Input: part model. Units: mm. Frame: model coordinates. A direction names the side the tool comes from. Give positions to 0.01 mm unless a question says otherwise; leave off trailing zeros. Order: outer loops, then holes, each group sorted by start corner. A loop starts at its lowest first (then second) coordinate and runs counter-clockwise, first axis right, second up. Notation, with made-up numbers: (-10.75, 43.25) - (8.25, 43.25) arc R19 ccw to (8.25, 60.25) - close; hole circle Ø6 at (-22.5, 83.25). An arc over 180 degrees is marked (long way). Answer in a Markdown table with one row per item. Add a question column.
1. Contact query for flat-ended pins moving along their axis: pin 1 (5.5 mm diameter, centred on x = -14.8, y = -14.8, fed in from -Z); pin 2 (10 mm diameter, centred on x = -7.5, z = -14.5, fed in from -Y); pin 3 (2 mm diameter, centred on x = 1.5, y = -8.5, fed in from +Z); pin 4 (0.5 mm diameter, centred on y = 5.5, z = 41, fed in from -X). Output: stop coordinate, or through.
2. Mould query, pull axis Y, two halves, no side actions, for faces 4 (the face through (0, 4.561, 36)), 5 (the face through (18.1, -18.14, 6.12)), 6 (the face through (16.9, 14.89, -29.26)). Classes: released by +Y, released by -Y, zero draft, split by the parting line, or undercut.
3. Access query for faces 1 (the face through (10.55, -15, 14)), 2 (the face through (-12, 14, 12.065)), 3 (the face through (1.588, 5, 37)). Directions: +Z, -Z, +X, -X, +Y, -Y. A direction counts if a zero-diameter tool reaches every point of the face in a straight line with its end or side. Return the directions, or none.
4. Section query D-D on y = 8. Return loops of the section in (x, z), and give its area (3 significant figures).
5. Section query A-A on x = 14.8. Count the separate pieces of the cut face and the enclosed holes in it, and give its area (3 significant figures).
6. Section query C-C on z = 47. Return loops of the section in (x, y), and give its area (3 significant figures).
7. Ray query, line 1 (X direction, y = -14.8, z = 5.25); line 2 (Y direction, x = 14.8, z = -27.75). Return the intervals inside material, ascending. Write a range as [from, to].
```python
from build123d import *

# Parameters (mm, degrees)
SKETCH1_W                      = 38.1
SKETCH1_H                      = 38.1
EXTRUDE1_DEPTH                 = 15.24
FILLET1_R                      = 3.175
SKETCH2_R                      = 6.35
EXTRUDE2_DEPTH                 = 38.1
CHAMFER1_SIZE                  = 1
SKETCH3_W                      = 3.175
SKETCH3_H                      = 3.175
EXTRUDE3_DEPTH                 = 35
FILLET2_R                      = 1.5875
M5X0_8_TAPPED_HOLE1_D          = 4.2
M5X0_8_TAPPED_HOLE1_DEPTH      = 14
M5X0_8_TAPPED_HOLE1_TIP        = 1.2618073
SKETCH7_R                      = 18.5
EXTRUDE4_DEPTH                 = 25.4
EXTRUDE5_DEPTH                 = 7.62
SKETCH9_W                      = 8.5
SKETCH9_H                      = 8.5
EXTRUDE7_DEPTH                 = 3.175
FILLET3_R                      = 1.5
SKETCH10_R                     = 2.5
EXTRUDE8_DEPTH                 = 12.065
M5X0_8_TAPPED_HOLE2_D          = 4.2
M5X0_8_TAPPED_HOLE3_AT_2_COUNT = 2
M5X0_8_TAPPED_HOLE3_AT_2_PITCH = 19.05
M5X0_8_TAPPED_HOLE3_AT_3_COUNT = 2
M5X0_8_TAPPED_HOLE3_AT_3_PITCH = 36.83
M5X0_8_TAPPED_HOLE3_AT_4_COUNT = 2
M5X0_8_TAPPED_HOLE3_AT_4_PITCH = 41.465062402


with BuildPart() as part:
    # Sketch1 → Extrude1 (new body)
    with BuildSketch(Plane.XY):
        Rectangle(SKETCH1_W, SKETCH1_H)
    extrude(amount=EXTRUDE1_DEPTH)

    # Fillet1
    fillet1_edges = [part.edges().sort_by_distance(p)[0] for p in [
        (19.05, -19.05, 7.62),
        (-19.05, -19.05, 7.62),
        (-19.05, 19.05, 7.62),
        (19.05, 19.05, 7.62),
    ]]
    fillet(fillet1_edges, radius=FILLET1_R)

    # Sketch2 → Extrude2 (add)
    with BuildSketch(Plane.XY.offset(15.24)):
        with Locations(Location((0, 0, 0), (0, 0, 180))):
            Circle(SKETCH2_R)
    extrude(amount=EXTRUDE2_DEPTH)

    # Chamfer1
    chamfer1_edges = [part.edges().sort_by_distance(p)[0] for p in [
        (6.35, 0, 53.34),
    ]]
    chamfer(chamfer1_edges, length=CHAMFER1_SIZE)

    # Sketch3 → Extrude3 (cut)
    with BuildSketch(Plane.XY.offset(53.34)):
        with Locations((0, 6.148361062)):
            Rectangle(SKETCH3_W, SKETCH3_H)
    extrude(amount=-EXTRUDE3_DEPTH, mode=Mode.SUBTRACT)

    # Fillet2
    fillet2_edges = [part.edges().sort_by_distance(p)[0] for p in [
        (1.5875, 5.354611062, 18.34),
        (-1.5875, 5.354611062, 18.34),
    ]]
    fillet(fillet2_edges, radius=FILLET2_R - 0.0001)  # a hair under: the kernel refuses the full size

    # M5x0.8 Tapped Hole1
    with Locations(Plane.XY.offset(53.34)):
        with Locations((0, 0)):
            Hole(M5X0_8_TAPPED_HOLE1_D / 2, depth=M5X0_8_TAPPED_HOLE1_DEPTH)
            with Locations((0, 0, -(M5X0_8_TAPPED_HOLE1_DEPTH + M5X0_8_TAPPED_HOLE1_TIP / 2))):  # 118° drill point
                Cone(0, M5X0_8_TAPPED_HOLE1_D / 2, M5X0_8_TAPPED_HOLE1_TIP, mode=Mode.SUBTRACT)

    # Sketch7 → Extrude4 (add)
    with BuildSketch(Plane(origin=(0, 0, 0), x_dir=(-1, 0, 0), z_dir=(0, 0, -1))):
        Circle(SKETCH7_R)
    extrude(amount=EXTRUDE4_DEPTH)

    # Sketch8 → Extrude5 (add)
    with BuildSketch(Plane(origin=(0, 0, -25.4), x_dir=(-1, 0, 0), z_dir=(0, 0, -1))):
        with BuildLine():
            Line((-15.875, -19.05), (15.875, -19.05))
            ThreePointArc((15.875, -19.05), (18.12006403, -18.12006403), (19.05, -15.875))
            Line((19.05, -15.875), (19.05, 15.875))
            ThreePointArc((19.05, 15.875), (18.12006403, 18.12006403), (15.875, 19.05))
            Line((15.875, 19.05), (-15.875, 19.05))
            ThreePointArc((-15.875, 19.05), (-18.12006403, 18.12006403), (-19.05, 15.875))
            Line((-19.05, 15.875), (-19.05, -15.875))
            ThreePointArc((-19.05, -15.875), (-18.12006403, -18.12006403), (-15.875, -19.05))
        make_face()
    extrude(amount=EXTRUDE5_DEPTH)

    # Sketch9 → Extrude7 (cut)
    with BuildSketch(Plane.XY.offset(15.24)):
        with Locations((-14.8, 14.8)):
            Rectangle(SKETCH9_W, SKETCH9_H)
        with Locations((14.8, 14.8)):
            Rectangle(SKETCH9_W, SKETCH9_H)
        with Locations((14.8, -14.8)):
            Rectangle(SKETCH9_W, SKETCH9_H)
        with Locations((-14.8, -14.8)):
            Rectangle(SKETCH9_W, SKETCH9_H)
    extrude(amount=-EXTRUDE7_DEPTH, mode=Mode.SUBTRACT)

    # Fillet3
    fillet3_edges = [part.edges().sort_by_distance(p)[0] for p in [
        (-19.05, 10.55, 13.6525),
        (-10.55, 19.05, 13.6525),
        (-10.55, 10.55, 13.6525),
        (10.55, 19.05, 13.6525),
        (19.05, 10.55, 13.6525),
        (10.55, 10.55, 13.6525),
        (19.05, -10.55, 13.6525),
        (10.55, -19.05, 13.6525),
        (10.55, -10.55, 13.6525),
        (-10.55, -19.05, 13.6525),
        (-19.05, -10.55, 13.6525),
        (-10.55, -10.55, 13.6525),
    ]]
    fillet(fillet3_edges, radius=FILLET3_R)

    # Sketch10 → Extrude8 (cut)
    with BuildSketch(Plane.XY.offset(12.065)):
        with Locations((-14.8, 14.8)):
            Circle(SKETCH10_R)
        with Locations(Location((-14.8, -14.8, 0), (0, 0, 32.271518342))):
            Circle(SKETCH10_R)
        with Locations((14.8, -14.8)):
            Circle(SKETCH10_R)
        with Locations(Location((14.8, 14.8, 0), (0, 0, 237.728481658))):
            Circle(SKETCH10_R)
    extrude(amount=-EXTRUDE8_DEPTH, mode=Mode.SUBTRACT)

    # M5x0.8 Tapped Hole2 (through all)
    with Locations(Plane.XY.offset(-25.4)):
        with Locations((-14.8, 14.8), (14.8, 14.8), (14.8, -14.8), (-14.8, -14.8)):
            Hole(M5X0_8_TAPPED_HOLE2_D / 2)

    # Sketch13 → M5x0.8 Tapped Hole3 (revolve, cut)
    with BuildSketch(Plane(origin=(-9.525, 19.05, -29.21), x_dir=(0, 0, 1), z_dir=(1, 0, 0))):
        Polygon((0, 0), (0, 8.8818073), (2.1, 7.62), (2.1, 0), align=None)
    m5x0_8_tapped_hole3 = revolve(axis=Axis((-9.525, 25.4, -29.21), (0, -1, 0)), mode=Mode.SUBTRACT)

    # M5x0.8 Tapped Hole3 at 2: M5x0.8 Tapped Hole3 ×2
    with Locations(*[(i * M5X0_8_TAPPED_HOLE3_AT_2_PITCH, 0, 0) for i in range(1, M5X0_8_TAPPED_HOLE3_AT_2_COUNT)]):
        add(m5x0_8_tapped_hole3, mode=Mode.SUBTRACT)

    # M5x0.8 Tapped Hole3 at 3: M5x0.8 Tapped Hole3 ×2
    with Locations(*[(0, 0, i * M5X0_8_TAPPED_HOLE3_AT_3_PITCH) for i in range(1, M5X0_8_TAPPED_HOLE3_AT_3_COUNT)]):
        add(m5x0_8_tapped_hole3, mode=Mode.SUBTRACT)

    # M5x0.8 Tapped Hole3 at 4: M5x0.8 Tapped Hole3 ×2
    with Locations(*[Vector(0.4594229188737666, 0, 0.8882176431559489) * (i * M5X0_8_TAPPED_HOLE3_AT_4_PITCH) for i in range(1, M5X0_8_TAPPED_HOLE3_AT_4_COUNT)]):
        add(m5x0_8_tapped_hole3, mode=Mode.SUBTRACT)

    # Mirror2: M5x0.8 Tapped Hole3 across plane
    add(m5x0_8_tapped_hole3.mirror(Plane.ZX), mode=Mode.SUBTRACT)

    # Mirror2 copy 1 sketch → Mirror2 copy 1 (revolve, cut)
    with BuildSketch(Plane(origin=(9.525, -19.05, -29.21), x_dir=(0, 0, 1), z_dir=(1, 0, 0))):
        Polygon((0, 0), (0, -8.8818073), (2.1, -7.62), (2.1, 0), align=None)
    revolve(axis=Axis((9.525, -25.4, -29.21), (0, -1, 0)), mode=Mode.SUBTRACT)

    # Mirror2 copy 2 sketch → Mirror2 copy 2 (revolve, cut)
    with BuildSketch(Plane(origin=(-9.525, -19.05, 7.62), x_dir=(0, 0, 1), z_dir=(1, 0, 0))):
        Polygon((0, 0), (0, -8.8818073), (2.1, -7.62), (2.1, 0), align=None)
    revolve(axis=Axis((-9.525, -25.4, 7.62), (0, -1, 0)), mode=Mode.SUBTRACT)

    # Mirror2 copy 3 sketch → Mirror2 copy 3 (revolve, cut)
    with BuildSketch(Plane(origin=(9.525, -19.05, 7.62), x_dir=(0, 0, 1), z_dir=(1, 0, 0))):
        Polygon((0, 0), (0, -8.8818073), (2.1, -7.62), (2.1, 0), align=None)
    revolve(axis=Axis((9.525, -25.4, 7.62), (0, -1, 0)), mode=Mode.SUBTRACT)


solid = part.part
```
Answer:
| question | item | result |
|---|---|---|
| 1 | pin 1 | stops at z = -33.02 |
| 1 | pin 2 | stops at y = -18.33 |
| 1 | pin 3 | stops at z = 15.24 |
| 1 | pin 4 | stops at x = -3.57 |
| 2 | face 4 | released by +Y |
| 2 | face 5 | released by -Y |
| 2 | face 6 | undercut |
| 3 | face 1 | +Z, +X, -Y |
| 3 | face 2 | +Z, -X, +Y |
| 3 | face 3 | +Z, +Y |
| 4 | outline | (-19.05, -33.02) - (19.05, -33.02) - (19.05, -25.4) - (16.68, -25.4) - (16.68, 0) - (19.05, 0) - (19.05, 15.24) - (-19.05, 15.24) - (-19.05, 0) - (-16.68, 0) - (-16.68, -25.4) - (-19.05, -25.4) - close |
| 4 | area | 1,720 mm² |
| 5 | separate pieces | 5 |
| 5 | enclosed holes | 0 |
| 5 | area | 1,200 mm² |
| 6 | outline | (-1.59, 4.56) - (-1.59, 6.15) arc R6.35 ccw (long way) to (1.59, 6.15) - (1.59, 4.56) - close; hole circle Ø4.2 at (0, 0) |
| 6 | area | 107 mm² |
| 7 | line 1 | x = [-19.05, -17.3], [-12.3, 12.3], [17.3, 19.05] |
| 7 | line 2 | y = [-19.05, -16.9], [-12.7, 12.7], [16.9, 19.05] |
